Build history of the part. All positions in model axes, mm. A direction names the side the tool comes from. Round coordinates to 2 decimals unless told otherwise and drop trailing zeros. Write each loop counter-clockwise with the first axis right and the second up, starting at its lowest first coordinate (ties: lowest second). Pieces come first, ordered by that corner, then holes. Notation, with made-up numbers: M 36.5,9 L 62.5,9 A27 ccw 62.5,48 Z; hole C 43,57 d4. An arc over 180 degrees is marked long. One line per item, written item: value. Start each with the question number.
```python
from build123d import *

# Parameters (mm, degrees)
SKETCH2_R           = 24
SKETCH2_R_2         = 12
BOSS_EXTRUDE2_DEPTH = 18
SKETCH3_R           = 24
SKETCH3_R_2         = 12
BOSS_EXTRUDE3_DEPTH = 18
BOSS_EXTRUDE4_DEPTH = 14
SKETCH6_R           = 12.5
BOSS_EXTRUDE5_DEPTH = 20
BOSS_EXTRUDE7_START = -18
BOSS_EXTRUDE7_DEPTH = 18
BOSS_EXTRUDE8_DEPTH = 18


with BuildPart() as part:
    # Sketch2 → Boss-Extrude2 (new body)
    with BuildSketch(Plane(origin=(0, 0, 0), x_dir=(1, 0, 0), z_dir=(0, 1, 0))):
        with Locations(Location((0, 0, 0), (0, 0, 270))):
            Circle(SKETCH2_R)
        with Locations(Location((0, 0, 0), (0, 0, 270))):
            Circle(SKETCH2_R_2, mode=Mode.SUBTRACT)
    extrude(amount=BOSS_EXTRUDE2_DEPTH)



with BuildPart() as body_2:
    # Sketch3 → Boss-Extrude3 (new body)
    with BuildSketch(Plane(origin=(0, 46, 0), x_dir=(1, 0, 0), z_dir=(0, 1, 0))):
        with Locations(Location((0, 0, 0), (0, 0, 270))):
            Circle(SKETCH3_R)
        with Locations(Location((0, 0, 0), (0, 0, 270))):
            Circle(SKETCH3_R_2, mode=Mode.SUBTRACT)
    extrude(amount=BOSS_EXTRUDE3_DEPTH)



with BuildPart() as body_3:
    # Sketch4 → Boss-Extrude4 (new, symmetric)
    with BuildSketch(Plane.XY):
        with BuildLine():
            Line((-24, 64), (-24, 46))
            ThreePointArc((-24, 46), (-38, 32), (-24, 18))
            Line((-24, 18), (-24, 0))
            ThreePointArc((-24, 0), (-56, 32), (-24, 64))
        make_face()
    extrude(amount=BOSS_EXTRUDE4_DEPTH, both=True)

    # Sketch5 → Revolve1 (revolve)
    with BuildSketch(Plane.XY, mode=Mode.PRIVATE) as revolve1_sk:
        with BuildLine():
            Line((-52.77498914, 46), (-128, 46))
            Line((-128, 46), (-128, 32))
            Line((-128, 32), (-56, 32))
            ThreePointArc((-56, 32), (-55.183326093, 39.183326093), (-52.77498914, 46))
        make_face()
    revolve(revolve1_sk.sketch.rotate(Axis((-128, 32, 0), (1, 0, 0)), 180), axis=Axis((-128, 32, 0), (1, 0, 0)))

    # Sketch6 → Boss-Extrude5 (add)
    with BuildSketch(Plane.ZY.offset(128)):
        with Locations(Location((0, 32, 0), (0, 0, 270))):
            Circle(SKETCH6_R)
    extrude(amount=BOSS_EXTRUDE5_DEPTH)


with BuildPart() as body_2_1:
    add(body_2.part)

    add(body_3.part)  # Boss-Extrude7 merges body 3
    # Sketch7 → Boss-Extrude7 (add)
    with BuildSketch(Plane(origin=(0, 64, 0), x_dir=(1, 0, 0), z_dir=(0, 1, 0)).offset(BOSS_EXTRUDE7_START)):
        with BuildLine():
            Line((-24, 14), (-19.49358869, 14))
            ThreePointArc((-19.49358869, 14), (-22.845635563, 7.353702178), (-24, 0))
            Line((-24, 0), (-24, 14))
        make_face()
    boss_extrude7 = extrude(amount=BOSS_EXTRUDE7_DEPTH)

    # Mirror1: Boss-Extrude7 across plane
    add(boss_extrude7.mirror(Plane.XY))


with BuildPart() as part_1:
    add(part.part)

    add(body_2_1.part)  # Boss-Extrude8 merges body 2
    # Sketch8 → Boss-Extrude8 (add)
    with BuildSketch(Plane.XZ):
        with BuildLine():
            Line((-24, 14), (-19.49358869, 14))
            ThreePointArc((-19.49358869, 14), (-22.845635563, 7.353702178), (-24, 0))
            Line((-24, 0), (-24, 14))
        make_face()
    boss_extrude8 = extrude(amount=-BOSS_EXTRUDE8_DEPTH)

    # Mirror2: Boss-Extrude8 across plane
    add(boss_extrude8.mirror(Plane.XY))


solid = part_1.part
```
Item 1: Drill centre lines: line 1 (Y direction, x = -2.5, z = -15); line 2 (X direction, y = 50.25, z = 0); line 3 (Z direction, x = -103.5, y = 31). Where is each one in solid material? Low to high.
Item 2: Cut at B-B, the plane z = -3. Write the cut outline in (x, y).
Item 3: Two-plate mould, pull along Y, no slides. Class faces 1 (the cylindrical face through (-42.64, 58.01, 0.2)), 2 (the flat face through (11, 18, -6)), 3 (the cylindrical face through (23.985, 54.874, 0.846)): pulls with the +Y half, pulls with the -Y half, needs draft (parallel to the pull), parting line crosses it, or undercut.
Item 4: Drop flat-ended pins along their axis: pin 1 (1.5 mm diameter, centred on x = -41, y = 8.5, fed in from +Z); pin 2 (6 mm diameter, centred on x = -31, z = 11.5, fed in from +Y); pin 3 (3 mm diameter, centred on x = -106, z = 4, fed in from +Y) (3 decimals); pin 4 (24 mm diameter, centred on x = -4, z = -2.5, fed in from +Y). Give the stop position or say it passes through.
Item 5: Cut at D-D, the plane z = 20. Write the cut outline in (x, y), plus the area to 3 significant figures.
Item 6: Which spindle directions (+Z, -Z, +X, -X, +Y, -Y) get a long thin tool onto all of the face, cutting with end or side? Do faces 4 (the flat face through (-42, 32, 14)), 5 (the cylindrical face through (-90.888, 45.986, -0.616)), 6 (the flat face through (-42, 32, -14)). Say none if no direction does.
Item 7: Cut at C-C, the plane y = 40. Write the cut outline in (x, z).
Item 8: Cut at A-A, the plane x = 0. Write the cut outline in (y, z).
Computed values:
1. line 1: y = 0 to 18, 46 to 64
1. line 2: x = -50.29 to -12, 12 to 24
1. line 3: z = -13.96 to 13.96
2. outline: M -148,19.87 L -128,19.87 L -128,18.33 L -52.93,18.33 A32 ccw -24,0 L -11.62,0 L -11.62,18 L -24,18 A14 cw -24,46 L -11.62,46 L -11.62,64 L -24,64 A32 ccw -52.88,45.78 L -128,45.67 L -128,44.13 L -148,44.13 Z; M 11.62,0 L 23.81,0 L 23.81,18 L 11.62,18 Z; M 11.62,46 L 23.81,46 L 23.81,64 L 11.62,64 Z
3. face 1: pulls with the +Y half
3. face 2: undercut
3. face 3: needs draft
4. pin 1: stops at z = 14
4. pin 2: stops at y = 63.75
4. pin 3: stops at y = 45.775
4. pin 4: stops at y = 64
5. outline: M -13.27,0 L 13.27,0 L 13.27,18 L -13.27,18 Z; M -13.27,46 L 13.27,46 L 13.27,64 L -13.27,64 Z
5. area: 955 mm2
6. face 4: +Z, -X, +Y, -Y
6. face 5: -X
6. face 6: -Z, -X, +Y, -Y
7. outline: M -148,-9.6 L -128,-9.6 L -128,-11.49 L -54.98,-11.49 L -54.98,-14 L -35.49,-14 L -35.49,14 L -54.98,14 L -54.98,11.49 L -128,11.49 L -128,9.6 L -148,9.6 Z
8. outline: M 0,-24 L 18,-24 L 18,-12 L 0,-12 Z; M 0,12 L 18,12 L 18,24 L 0,24 Z; M 46,-24 L 64,-24 L 64,-12 L 46,-12 Z; M 46,12 L 64,12 L 64,24 L 46,24 Z
